```python
from build123d import *

# Parameters (mm, degrees)
SKETCH2_R           = 2
SKETCH2_R_2         = 1.999999991
BOSS_EXTRUDE1_DEPTH = 5.588
SKETCH7_R           = 2.032
CUT_EXTRUDE1_DEPTH  = 5.588
CUT_EXTRUDE2_DEPTH  = 226.492641696


with BuildPart() as part:
    # Sketch2 → Boss-Extrude1 (new body)
    with BuildSketch(Plane(origin=(0, 0, 0), x_dir=(1, 0, 0), z_dir=(0, 1, 0))):
        with BuildLine():
            ThreePointArc((17.295902343, -29.323452593), (16.73639375, -27.733089808), (15.304363929, -26.843373987))
            Line((15.304363929, -26.843373987), (13.284423018, -26.396670406))
            ThreePointArc((13.284423018, -26.396670406), (11.420627025, -25.189010374), (10.804170553, -23.055431298))
            Line((10.804170553, -23.055431298), (12.5603, 0))
            ThreePointArc((12.5603, 0), (0.640974044, 12.543934326), (-12.49487995, 1.28027775))
            Line((-12.49487995, 1.28027775), (-16.496770465, -37.776201638))
            ThreePointArc((-16.496770465, -37.776201638), (-16.50669046, -37.90548449), (-16.51, -38.035105126))
            Line((-16.51, -38.035105126), (-16.51, -220.313887427))
            ThreePointArc((-16.51, -220.313887427), (-12.970187584, -224.665744552), (-7.988667969, -222.086327038))
            Line((-7.988667969, -222.086327038), (16.979901226, -164.662549258))
            ThreePointArc((16.979901226, -164.662549258), (17.216065593, -163.919190378), (17.295902343, -163.143315306))
            Line((17.295902343, -163.143315306), (17.295902343, -29.323452593))
        make_face()
        with Locations(Location((-11.43, -219.075, 0), (0, 0, 270))):
            Circle(SKETCH2_R, mode=Mode.SUBTRACT)
        with Locations(Location((-11.43, -212.725, 0), (0, 0, 270))):
            Circle(SKETCH2_R, mode=Mode.SUBTRACT)
        with Locations(Location((-11.43, -206.375, 0), (0, 0, 270))):
            Circle(SKETCH2_R, mode=Mode.SUBTRACT)
        with Locations(Location((-11.43, -200.025, 0), (0, 0, 270))):
            Circle(SKETCH2_R, mode=Mode.SUBTRACT)
        with BuildLine():
            ThreePointArc((7.135902343, -161.395796446), (8.023611961, -164.633987883), (10.438542905, -166.966801782))
            Line((10.438542905, -166.966801782), (-0.894016375, -193.029903785))
            ThreePointArc((-0.894016375, -193.029903785), (-2.665854515, -194.495144898), (-4.89449504, -193.929898651))
            Line((-4.89449504, -193.929898651), (-11.831146076, -187.869646091))
            ThreePointArc((-11.831146076, -187.869646091), (-12.472607947, -187.007278248), (-12.7, -185.95682859))
            Line((-12.7, -185.95682859), (-12.7, -146.861981888))
            ThreePointArc((-12.7, -146.861981888), (-11.955224829, -145.705677915), (-10.594426962, -145.905573138))
            Line((-10.594426962, -145.905573138), (7.135902343, -161.395796446))
        make_face(mode=Mode.SUBTRACT)
        with BuildLine():
            ThreePointArc((12.215902343, -151.955842791), (10.785297541, -152.261664921), (9.418398214, -152.782955151))
            Line((9.418398214, -152.782955151), (-10.962292152, -134.977225798))
            ThreePointArc((-10.962292152, -134.977225798), (-12.245215894, -133.252490112), (-12.7, -131.151590796))
            Line((-12.7, -131.151590796), (-12.7, -90.4875))
            ThreePointArc((-12.7, -90.4875), (-11.765673597, -90.432318214), (-10.844338135, -90.267540106))
            Line((-10.844338135, -90.267540106), (11.513275375, -128.23323342))
            ThreePointArc((11.513275375, -128.23323342), (12.037098881, -129.475107855), (12.215902343, -130.811024207))
            Line((12.215902343, -130.811024207), (12.215902343, -151.955842791))
        make_face(mode=Mode.SUBTRACT)
        with Locations(Location((13.485902343, -161.395796446, 0), (0, 0, 270))):
            Circle(SKETCH2_R, mode=Mode.SUBTRACT)
        with BuildLine():
            Line((-10.16, -41.91), (2.838491406, -41.91))
            ThreePointArc((2.838491406, -41.91), (3.914572403, -42.505500417), (3.981509018, -43.733543799))
            Line((3.981509018, -43.733543799), (-11.055993219, -74.784618621))
            ThreePointArc((-11.055993219, -74.784618621), (-11.873503915, -74.655646925), (-12.7, -74.6125))
            Line((-12.7, -74.6125), (-12.7, -44.45))
            ThreePointArc((-12.7, -44.45), (-11.956051224, -42.653948776), (-10.16, -41.91))
        make_face(mode=Mode.SUBTRACT)
        with BuildLine():
            ThreePointArc((-9.886442157, -38.1), (-11.771808813, -37.262055396), (-12.413212622, -35.301096512))
            Line((-12.413212622, -35.301096512), (-9.81475239, -9.941405108))
            ThreePointArc((-9.81475239, -9.941405108), (-3.431386466, -13.542026692), (3.896359547, -13.415635739))
            Line((3.896359547, -13.415635739), (2.194931831, -35.752912681))
            ThreePointArc((2.194931831, -35.752912681), (1.388767881, -37.42300808), (-0.337731726, -38.1))
            Line((-0.337731726, -38.1), (-9.886442157, -38.1))
        make_face(mode=Mode.SUBTRACT)
        with BuildLine():
            ThreePointArc((3.111707299, -3.622128204), (-4.505881672, 1.581001391), (4.69270869, 0.883753468))
            Line((4.69270869, 0.883753468), (3.111707299, -3.622128204))
        make_face(mode=Mode.SUBTRACT)
        with BuildLine():
            ThreePointArc((-8.804706991, -86.222769023), (-8.262040897, -82.55), (-8.804706991, -78.877230977))
            Line((-8.804706991, -78.877230977), (8.75092063, -42.626456201))
            ThreePointArc((8.75092063, -42.626456201), (9.219438659, -42.103919003), (9.893938242, -41.91))
            Line((9.893938242, -41.91), (10.945902343, -41.91))
            ThreePointArc((10.945902343, -41.91), (11.843927955, -42.281974388), (12.215902343, -43.18))
            Line((12.215902343, -43.18), (12.215902343, -62.618124667))
            ThreePointArc((12.215902343, -62.618124667), (6.906756389, -72.428110561), (13.516748759, -81.413145613))
            Line((13.516748759, -81.413145613), (13.516748759, -119.431411199))
            ThreePointArc((13.516748759, -119.431411199), (12.599191369, -120.688899116), (11.152950849, -120.113072943))
            Line((11.152950849, -120.113072943), (-8.804706991, -86.222769023))
        make_face(mode=Mode.SUBTRACT)
        with Locations(Location((13.485902343, -38.1, 0), (0, 0, 270))):
            Circle(SKETCH2_R_2, mode=Mode.SUBTRACT)
    extrude(amount=BOSS_EXTRUDE1_DEPTH)

    # Sketch7 → Cut-Extrude1 (cut)
    with BuildSketch(Plane(origin=(0, 5.588, 0), x_dir=(1, 0, 0), z_dir=(0, 1, 0))):
        with Locations(Location((12.215902343, -72.362149281, 0), (0, 0, 270))):
            Circle(SKETCH7_R)
    extrude(amount=-CUT_EXTRUDE1_DEPTH, mode=Mode.SUBTRACT)

    # Sketch8 → Cut-Extrude2 (cut, through all)
    with BuildSketch(Plane(origin=(0, 5.588, 0), x_dir=(1, 0, 0), z_dir=(0, 1, 0))):
        with BuildLine():
            Line((1.104680914, 5.054256967), (-2.867487033, 4.306199197))
            ThreePointArc((-2.867487033, 4.306199197), (-3.806203053, 4.430543784), (-3.824774473, 3.483810218))
            Line((-3.824774473, 3.483810218), (-5.163021415, -0.330217017))
            ThreePointArc((-5.163021415, -0.330217017), (-5.740064996, -1.080996644), (-4.929455388, -1.570446748))
            Line((-4.929455388, -1.570446748), (-2.295534382, -4.636416214))
            ThreePointArc((-2.295534382, -4.636416214), (-1.933861943, -5.511540428), (-1.104680914, -5.054256967))
            Line((-1.104680914, -5.054256967), (2.867487033, -4.306199197))
            ThreePointArc((2.867487033, -4.306199197), (3.806203053, -4.430543784), (3.824774473, -3.483810218))
            Line((3.824774473, -3.483810218), (5.163021415, 0.330217017))
            ThreePointArc((5.163021415, 0.330217017), (5.740064996, 1.080996644), (4.929455388, 1.570446748))
            Line((4.929455388, 1.570446748), (2.295534382, 4.636416214))
            ThreePointArc((2.295534382, 4.636416214), (1.933861943, 5.511540428), (1.104680914, 5.054256967))
        make_face()
    extrude(amount=-CUT_EXTRUDE2_DEPTH, mode=Mode.SUBTRACT)


solid = part.part
```
Input: part model. Units: mm. Frame: model coordinates. A direction names the side the tool comes from. Round coordinates to 2 decimals unless told otherwise and drop trailing zeros. Loops run counter-clockwise (first coordinate to the right, second up) from the corner with the lowest first, then second, coordinate; pieces in that order, holes last. Notation, with made-up numbers: M -33,61 L 16,61 A25 ccw 16,90 Z; hole C 69,45.5 d11. An arc over 180 degrees is marked long. Answer in a Markdown table with one row per item. Add a question column.
1. Ray query, probe 1 along Z at (x, y) = (-6.5, 2.75); probe 2 along X at (y, z) = (2.75, 37.5); probe 3 along Z at (x, y) = (-7, 2.3). Return the intervals inside material, ascending.
2. Contact query for flat-ended pins moving along their axis: pin 1 (0.8 mm diameter, centred on x = 10.5, y = 4, fed in from +Z); pin 2 (1.5 mm diameter, centred on y = 5, z = 193, fed in from +X); pin 3 (2 mm diameter, centred on x = 7, y = 4.5, fed in from +Z). Output: stop coordinate, or through.
3. Mould query, pull axis X, two halves, no side actions, for faces 3 (the face through (-12.2, 2.75, 201.87)), 4 (the face through (0, 0, 104)), 5 (the face through (0.908, 2.755, -12.527)). Classes: released by +X, released by -X, zero draft, split by the parting line, or undercut.
4. Set-up query: faces 1 (the face through (0, 5.588, 104)), 2 (the face through (-3.43, 2.75, 59.04)). Return all of +Z, -Z, +X, -X, +Y, -Y with unobstructed straight access to the full face (end or side cutting, diameter ignored); none if empty.
5. Section C-C (z = 113). Output: boundary loops of the cut face in (x, y), and give its area (3 significant figures).
6. Section B-B (z = 84). Output: boundary loops of the cut face in (x, y).
7. Section A-A (z = 49.5). Output: boundary loops of the cut face in (x, y), and give its area (3 significant figures).
8. Section D-D (y = 3.4). Give the number of separate pieces and of enclosed holes in the cut face, and give its area (3 significant figures).
Values follow:
| question | item | result |
|---|---|---|
| 1 | probe 1 | -10.75 to 12.37, 38.1 to 41.91, 65.38 to 74.12, 90.14 to 97.64, 138.88 to 149.48, 192.53 to 218.66 |
| 1 | probe 2 | -16.47 to -11.53, 1.3 to 11.58, 15.39 to 17.3 |
| 1 | probe 3 | -10.43 to 12.09, 38.1 to 41.91, 66.41 to 75.15, 89.29 to 96.8, 138.44 to 149.05, 192.09 to 219.81 |
| 2 | pin 1 | z = 180.49 |
| 2 | pin 2 | x = 4.98 |
| 2 | pin 3 | z = 189.91 |
| 3 | face 3 | undercut |
| 3 | face 4 | zero draft |
| 3 | face 5 | split by the parting line |
| 4 | face 1 | +Z, -Z, +X, -X, +Y |
| 4 | face 2 | +Y, -Y |
| 5 | outline | M -16.51,0 L -12.7,0 L -12.7,5.59 L -16.51,5.59 Z; M 2.54,0 L 6.96,0 L 6.96,5.59 L 2.54,5.59 Z; M 13.52,0 L 17.3,0 L 17.3,5.59 L 13.52,5.59 Z |
| 5 | area | 67.1 mm^2 |
| 6 | outline | M -16.51,0 L -8.35,0 L -8.35,5.59 L -16.51,5.59 Z; M 13.52,0 L 17.3,0 L 17.3,5.59 L 13.52,5.59 Z |
| 7 | outline | M -16.51,0 L -12.7,0 L -12.7,5.59 L -16.51,5.59 Z; M 1.19,0 L 5.42,0 L 5.42,5.59 L 1.19,5.59 Z; M 12.22,0 L 17.3,0 L 17.3,5.59 L 12.22,5.59 Z |
| 7 | area | 73.3 mm^2 |
| 8 | separate pieces | 1 |
| 8 | enclosed holes | 13 |
| 8 | area | 3,400 mm^2 |
